Verification items for the finished model (mm, model axes). A direction names the side the tool comes from. Give positions to 0.01 mm unless a question says otherwise; leave off trailing zeros. Loops run counter-clockwise (first coordinate to the right, second up) from the corner with the lowest first, then second, coordinate; pieces in that order, holes last. Notation, with made-up numbers: (44.5, 0.5) -> (75.5, 0.5) arc R14 ccw to (75.5, 19.5) -> close; hole circle Ø5 at (64, -29). An arc over 180 degrees is marked (long way). Answer in a Markdown table with one row per item. Add a question column.
Q1. Section check B-B on y = 29.5. Enter the section's corners in (x, z), and give its area (3 significant figures).
Q2. Section check C-C on x = 25.5. Enter the section's corners in (y, z).
Q3. Set-up check for faces 1 (the face through (35, 34.2, 6)), 2 (the face through (4.5, 16, -1)), 3 (the face through (8, 14.75, -1)), 4 (the face through (8.2, 1.7, 0.8)), 5 (the face through (35, 22.2, 6)): record each of +Z, -Z, +X, -X, +Y, -Y from which the full face is reachable in a straight line by a thin tool's end or side.
Q4. Release check for a two-part mould opening along X. For faces 6 (the face through (4, 26, 4)), 7 (the face through (40, 6, -6)), 8 (the face through (22, 31, 4)) record: pulls with the +X half, pulls with the -X half, needs draft (parallel to the pull), parting line crosses it, or undercut.
Q5. Gauge pin test, flat ends, axial feed: P1, Ø1, axis at x = 37, z = -4.5, coming from the +Y side; P2, Ø13.5, axis at x = 23.5, y = 21.5, coming from the -Z side; P3, Ø3, axis at x = 7, z = -9, coming from the -Y side; P4, Ø12, axis at x = 31, y = 14.5, coming from the -Z side. Record the tip position at first contact, or that the pin passes through.
Q6. Section check A-A on z = -6. Enter the section's corners in (x, y), and give its area (3 significant figures).
Q7. Material ranges on probe 1 along X at (y, z) = (7.5, -5.5); probe 2 along Z at (x, y) = (22, 25); probe 3 along Y at (x, z) = (33.5, 5), recorded low to high.
Q8. Section check D-D on y = 4. Enter the section's corners in (x, z), and give its area (3 significant figures).
```python
from build123d import *

# Parameters (mm, degrees)
EXTRUDE1_DEPTH  = 1.6
SKETCH3_W       = 6
SKETCH3_H       = 2
EXTRUDE3_DEPTH  = 2.5
SKETCH4_W       = 10
SKETCH4_H       = 10
EXTRUDE4_DEPTH  = 12
SKETCH6_W       = 7
SKETCH6_H       = 7
EXTRUDE5_DEPTH  = 5.8
SKETCH8_R       = 0.8
EXTRUDE7_DEPTH  = 3.81
SKETCH9_W       = 6.3
SKETCH9_H       = 6.3
EXTRUDE8_DEPTH  = 5.8
FILLET1_R       = 3
SKETCH10_W      = 12
SKETCH10_H      = 12
EXTRUDE9_DEPTH  = 8
SKETCH11_W      = 6.2
SKETCH11_H      = 6.7
EXTRUDE10_DEPTH = 2.4


with BuildPart() as part:
    # Sketch1 → Extrude1 (new body)
    with BuildSketch(Plane.XY):
        Polygon((41.5, 3.4), (38.1, 0), (9.9, 0), (6.5, 3.4), (6.5, 10), (0, 10), (0, 40), (3, 40), (3, 47), (9, 47), (9, 50), (45, 50), (45, 15), (41.5, 15), align=None)
    extrude(amount=EXTRUDE1_DEPTH)

    # Sketch3 → Extrude3 (add)
    with BuildSketch(Plane(origin=(0, 0, 0), x_dir=(-1, 0, 0), z_dir=(0, 0, -1))):
        with Locations((-7.5, 45.25)):
            Rectangle(SKETCH3_W, SKETCH3_H)
        with Locations((-7.5, 15.75)):
            Rectangle(SKETCH3_W, SKETCH3_H)
    extrude(amount=EXTRUDE3_DEPTH)

    # Sketch4 → Extrude4 (add)
    with BuildSketch(Plane(origin=(0, 0, 0), x_dir=(-1, 0, 0), z_dir=(0, 0, -1))):
        with Locations((-35, 6.2)):
            Rectangle(SKETCH4_W, SKETCH4_H)
        with Locations((-24, 6.2)):
            Rectangle(SKETCH4_W, SKETCH4_H)
        with Locations((-13, 6.2)):
            Rectangle(SKETCH4_W, SKETCH4_H)
    extrude(amount=EXTRUDE4_DEPTH)

    # Sketch6 → Extrude5 (add)
    with BuildSketch(Plane.XY.offset(1.6)):
        with Locations((4.5, 29.5)):
            Rectangle(SKETCH6_W, SKETCH6_H)
    extrude(amount=EXTRUDE5_DEPTH)

    # Sketch8 → Extrude7 (add)
    with BuildSketch(Plane(origin=(1, 0, 4), x_dir=(0, 0, -1), z_dir=(1, 0, 0))):
        with Locations(Location((-0.5, 29.5, 0), (0, 0, 90))):
            Circle(SKETCH8_R)
    extrude(amount=-EXTRUDE7_DEPTH)

    # Sketch9 → Extrude8 (add)
    with BuildSketch(Plane.XY.offset(1.6)):
        with Locations((23.15, 34.15)):
            Rectangle(SKETCH9_W, SKETCH9_H)
    extrude(amount=EXTRUDE8_DEPTH)

    # Fillet1
    fillet1_edges = [part.edges().sort_by_distance(p)[0] for p in [
        (26.3, 31, 4.5),
        (26.3, 37.3, 4.5),
    ]]
    fillet(fillet1_edges, radius=FILLET1_R)

    # Sketch10 → Extrude9 (add)
    with BuildSketch(Plane.XY.offset(1.6)):
        with Locations((35, 28.2)):
            Rectangle(SKETCH10_W, SKETCH10_H)
    extrude(amount=EXTRUDE9_DEPTH)

    # Sketch11 → Extrude10 (add)
    with BuildSketch(Plane.XY.offset(1.6)):
        with Locations((34.4, 17.05)):
            Rectangle(SKETCH11_W, SKETCH11_H)
    extrude(amount=EXTRUDE10_DEPTH)


solid = part.part
```
Taken from the geometry:
| question | item | result |
|---|---|---|
| 1 | outline | (-2.81, 3.7) -> (1, 3.7) -> (1, 1.6) -> (0, 1.6) -> (0, 0) -> (45, 0) -> (45, 1.6) -> (41, 1.6) -> (41, 9.6) -> (29, 9.6) -> (29, 1.6) -> (8, 1.6) -> (8, 7.4) -> (1, 7.4) -> (1, 5.3) -> (-2.81, 5.3) -> close |
| 1 | area | 215 mm² |
| 2 | outline | (0, 0) -> (1.2, 0) -> (1.2, -12) -> (11.2, -12) -> (11.2, 0) -> (50, 0) -> (50, 1.6) -> (36.34, 1.6) -> (36.34, 7.4) -> (31.96, 7.4) -> (31.96, 1.6) -> (0, 1.6) -> close |
| 3 | face 1 | +Z, +X, +Y |
| 3 | face 2 | -Z, -X, +Y, -Y |
| 3 | face 3 | -Z, +X, -X |
| 3 | face 4 | +Z, -X, -Y |
| 3 | face 5 | +Z, +X, -X |
| 4 | face 6 | needs draft |
| 4 | face 7 | pulls with the +X half |
| 4 | face 8 | undercut |
| 5 | P1 | stops at y = 11.2 |
| 5 | P2 | stops at z = 0 |
| 5 | P3 | stops at y = 1.2 |
| 5 | P4 | stops at z = -12 |
| 6 | outline | (8, 1.2) -> (18, 1.2) -> (18, 11.2) -> (8, 11.2) -> close; (19, 1.2) -> (29, 1.2) -> (29, 11.2) -> (19, 11.2) -> close; (30, 1.2) -> (40, 1.2) -> (40, 11.2) -> (30, 11.2) -> close |
| 6 | area | 300 mm² |
| 7 | probe 1 | x = 8 to 18, 19 to 29, 30 to 40 |
| 7 | probe 2 | z = 0 to 1.6 |
| 7 | probe 3 | y = 22.2 to 34.2 |
| 8 | outline | (6.5, 0) -> (8, 0) -> (8, -12) -> (18, -12) -> (18, 0) -> (19, 0) -> (19, -12) -> (29, -12) -> (29, 0) -> (30, 0) -> (30, -12) -> (40, -12) -> (40, 0) -> (41.5, 0) -> (41.5, 1.6) -> (6.5, 1.6) -> close |
| 8 | area | 416 mm² |
